CAD build for the part. Positions are in the model's coordinates, mm. A direction names the side the tool comes from. Coordinates: 2 decimals unless noted, no trailing zeros. Loops run counter-clockwise (first coordinate to the right, second up) from the corner with the lowest first, then second, coordinate; pieces in that order, holes last.
1) Wall check: line 1 along Z through (x, y) = (21, 27.5); line 2 along Y through (x, z) = (20, 40.5); line 3 along Y through (x, z) = (12.5, 50). Give the ranges that are in metal, low to high.
2) Which spindle directions (+Z, -Z, +X, -X, +Y, -Y) get a long thin tool onto all of the face, cutting with end or side? Do faces 4 (the flat face through (11, 18, 55.88)), 5 (the cylindrical face through (26.53, 64.59, 44.36)), 6 (the flat face through (23, 31, 36.83)), 7 (the cylindrical face through (22.1, 12.4, 61.5)), 8 (the cylindrical face through (0.724, 6.887, 0.764)). Say none if no direction does.
3) Saw through at C-C, the plane x = 4. Write the cut outline in (y, z), and give its area (3 significant figures).
4) Saw through at A-A, the plane z = 53. Write the cut outline in (x, y), and give its area (3 significant figures).
5) Saw through at D-D, the plane z = 45.5. Write the cut outline in (x, y).
6) Two-plate mould, pull along Z, no slides. Class faces 1 (the cylindrical face through (30.05, 25.503, 0.764)), 2 (the cylindrical face through (11.59, 0.724, 61.466)), 3 (the flat face through (21, 86.954, 45)): +Z half, -Z half, draft (parallel to the pull), parting line (faces both ways), or undercut.
7) Pin check, flat tips, straight feed: pin 1 Ø5 at (y, z) = (33, 25.5) entering from +X; pin 2 Ø1.2 at (x, z) = (21, 45.5) entering from +Y; pin 3 Ø8 at (x, y) = (17, 72.5) entering from +Z. Stop position of each tip, or through.
8) Saw through at B-B, the plane y = 32. Write the cut outline in (x, z).
```python
from build123d import *

# Parameters (mm, degrees)
BOSS_EXTRUDE1_DEPTH = 55.88
SKETCH2_W           = 22.86
SKETCH2_H           = 29.69248518
BOSS_EXTRUDE2_DEPTH = 6.35
BOSS_EXTRUDE3_DEPTH = 55.88
CUT_EXTRUDE1_DEPTH  = 55.88
BOSS_EXTRUDE5_DEPTH = 19.05
BOSS_EXTRUDE6_DEPTH = 19.05
SKETCH8_R           = 2.8575
CUT_EXTRUDE2_DEPTH  = 4.085289
SKETCH9_R           = 5.55625
BOSS_EXTRUDE7_DEPTH = 64.262
SKETCH11_R          = 1.999996
CUT_EXTRUDE3_DEPTH  = 6.99999997
BOSS_EXTRUDE8_DEPTH = 6.35
BOSS_EXTRUDE9_DEPTH = 6.35
FILLET3_R           = 2.54


with BuildPart() as part:
    # Sketch1 → Boss-Extrude1 (new body)
    with BuildSketch(Plane.XY):
        Polygon((0, 0), (22.86, 0), (22.86, 5.08), (0, 13.97), align=None)
    extrude(amount=BOSS_EXTRUDE1_DEPTH)

    # Sketch2 → Boss-Extrude2 (add)
    with BuildSketch(Plane.XY.offset(55.88)):
        with Locations((11.43, 14.84624259)):
            Rectangle(SKETCH2_W, SKETCH2_H)
    extrude(amount=BOSS_EXTRUDE2_DEPTH)

    # Sketch3 → Boss-Extrude3 (add)
    with BuildSketch(Plane(origin=(0, 0, 55.88), x_dir=(-1, 0, 0), z_dir=(0, 0, -1))):
        Polygon((-22.86, 29.69248518), (0, 29.69248518), (-30.774794254, 17.724509637), (-30.774794254, 29.69248518), align=None)
    extrude(amount=BOSS_EXTRUDE3_DEPTH)

    # Sketch5 → Cut-Extrude1 (cut)
    with BuildSketch(Plane(origin=(0, 0, 0), x_dir=(-1, 0, 0), z_dir=(0, 0, -1))):
        Polygon((-30.774794254, 22.107844851), (-11.271433408, 29.69248518), (-30.774794254, 29.69248518), align=None)
    extrude(amount=-CUT_EXTRUDE1_DEPTH, mode=Mode.SUBTRACT)

    # Sketch7 → Boss-Extrude6 (add)
    with BuildSketch(Plane.XY.offset(55.88)):
        Polygon((30.774794254, 22.107844851), (30.774794254, 29.69248518), (11.271433408, 29.69248518), align=None)
    extrude(amount=-BOSS_EXTRUDE6_DEPTH)

    # Sketch8 → Cut-Extrude2 (cut)
    with BuildSketch(Plane(origin=(11.510866943, 29.599372139, 0), x_dir=(0.9320046715412958, -0.36244626115494866, 0), z_dir=(0.36244626115494866, 0.9320046715412958, 0))):
        with Locations(Location((13.963299783, -27.94, 0), (0, 0, 180))):
            Circle(SKETCH8_R)
    extrude(amount=-CUT_EXTRUDE2_DEPTH, mode=Mode.SUBTRACT)



with BuildPart() as body_2:
    # Sketch6 → Boss-Extrude5 (new body)
    with BuildSketch(Plane(origin=(0, 0, 0), x_dir=(-1, 0, 0), z_dir=(0, 0, -1))):
        Polygon((-30.774794254, 29.69248518), (-30.774794254, 22.107844851), (-11.271433408, 29.69248518), align=None)
    extrude(amount=-BOSS_EXTRUDE5_DEPTH)


with BuildPart() as part_1:
    add(part.part)

    add(body_2.part)  # Boss-Extrude7 merges body 2
    # Sketch9 → Boss-Extrude7 (add)
    with BuildSketch(Plane(origin=(0, 29.69248518, 0), x_dir=(1, 0, 0), z_dir=(0, 1, 0))):
        with Locations(Location((21.023113831, -10.795, 0), (0, 0, 270))):
            Circle(SKETCH9_R)
        with Locations(Location((21.023113831, -45.085, 0), (0, 0, 270))):
            Circle(SKETCH9_R)
    extrude(amount=BOSS_EXTRUDE7_DEPTH)

    # Sketch11 → Cut-Extrude3 (cut)
    with BuildSketch(Plane(origin=(0, 93.95448518, 0), x_dir=(1, 0, 0), z_dir=(0, 1, 0))):
        with Locations(Location((21.023113831, -10.795, 0), (0, 0, 270))):
            Circle(SKETCH11_R)
        with Locations(Location((21.023113831, -45.085, 0), (0, 0, 270))):
            Circle(SKETCH11_R)
    extrude(amount=-CUT_EXTRUDE3_DEPTH, mode=Mode.SUBTRACT)

    # Sketch12 → Boss-Extrude8 (add)
    with BuildSketch(Plane.XY.offset(55.88)):
        Polygon((22.86, 29.69248518), (30.774794254, 29.69248518), (30.774794254, 17.724509637), (22.86, 20.80248518), align=None)
    extrude(amount=BOSS_EXTRUDE8_DEPTH)

    # Sketch14 → Boss-Extrude9 (add)
    with BuildSketch(Plane(origin=(0, 29.69248518, 0), x_dir=(1, 0, 0), z_dir=(0, 1, 0))):
        Polygon((0, 0), (0, -62.23), (30.774794254, -62.23), (30.774794254, -36.83), (11.271433408, -36.83), (11.271433408, -19.05), (30.774794254, -19.05), (30.774794254, 0), align=None)
    extrude(amount=BOSS_EXTRUDE9_DEPTH)

    # Fillet3
    fillet3_edges = [part_1.edges().sort_by_distance(p)[0] for p in [
        (0, 18.02124259, 62.23),
        (15.387397127, 36.04248518, 62.23),
        (30.774794254, 26.883497409, 0),
        (30.774794254, 26.883497409, 62.23),
        (26.817397127, 19.263497409, 62.23),
        (22.86, 10.40124259, 62.23),
        (11.43, 0, 62.23),
        (0, 6.985, 0),
        (15.387397127, 36.04248518, 0),
        (0, 36.04248518, 31.115),
        (30.774794254, 36.04248518, 49.53),
        (30.774794254, 36.04248518, 9.525),
    ]]
    fillet(fillet3_edges, radius=FILLET3_R)


solid = part_1.part
```
Data:
1. line 1: z = 0 to 19.05, 36.83 to 62.23
1. line 2: y = 0 to 6.19, 21.91 to 93.95
1. line 3: y = 0 to 9.11, 24.83 to 36.04
2. face 4: -Z
2. face 5: +Y
2. face 6: +X, +Y
2. face 7: +Z, -Y
2. face 8: -Z, -X, -Y
3. outline: (0, 0) - (12.41, 0) - (12.41, 55.88) - (28.14, 55.88) - (28.14, 0) - (33.5, 0) arc R2.54 ccw to (36.04, 2.54) - (36.04, 59.69) arc R2.54 ccw to (33.5, 62.23) - (2.54, 62.23) arc R2.54 ccw to (0, 59.69) - close
3. area: 1,360 mm2
4. outline: (0, 0) - (22.86, 0) - (22.86, 5.08) - (0, 13.97) - close; (0, 29.69) - (30.77, 17.72) - (30.77, 33.5) arc R2.54 ccw to (28.23, 36.04) - (2.54, 36.04) arc R2.54 ccw to (0, 33.5) - close
4. area: 595 mm2
5. outline: (0, 0) - (22.86, 0) - (22.86, 5.08) - (0, 13.97) - close; (0, 29.69) - (30.77, 17.72) - (30.77, 33.5) arc R2.54 ccw to (28.23, 36.04) - (26.56, 36.04) - (26.56, 93.95) - (22.98, 93.95) - (22.98, 86.95) - (19.07, 86.95) - (19.07, 93.95) - (15.48, 93.95) - (15.48, 36.04) - (2.54, 36.04) arc R2.54 ccw to (0, 33.5) - close
6. face 1: -Z half
6. face 2: +Z half
6. face 3: undercut
7. pin 1: stops at x = 11.27
7. pin 2: stops at y = 86.95
7. pin 3: stops at z = 50.64
8. outline: (0, 0) - (28.23, 0) arc R2.54 ccw to (30.77, 2.54) - (30.77, 19.05) - (11.27, 19.05) - (11.27, 36.83) - (30.77, 36.83) - (30.77, 59.69) arc R2.54 ccw to (28.23, 62.23) - (2.54, 62.23) arc R2.54 ccw to (0, 59.69) - close
